For this review, take the finished solid that the model builds, in its own axes (mm). Face numbers are marked on the shaded views. A direction names the side the tool comes from. Round coordinates to 2 decimals unless told otherwise and drop trailing zeros. Write each loop counter-clockwise with the first axis right and the second up, starting at its lowest first coordinate (ties: lowest second). Pieces come first, ordered by that corner, then holes. Notation, with made-up numbers: (-10, 58) -> (20, 58) arc R13 cw to (20, 73) -> close; hole circle Ø3 at (-23.75, -12). An arc over 180 degrees is marked (long way). Answer in a Markdown table with one row per item.
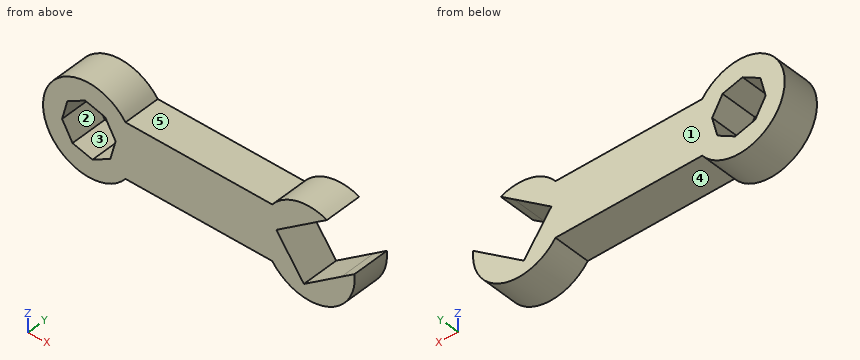
from build123d import *

# Parameters (mm, degrees)
F1_DEPTH = 25.4


with BuildPart() as f1:
    # F0 (on Front) → F1 (new body)
    with BuildSketch(Plane.XZ):
        with BuildLine():
            ThreePointArc((-50.790703, -19.05), (-46.070008, -10.040232), (-44.440703, 0))
            ThreePointArc((-44.440703, 0), (-46.070008, 10.040232), (-50.790703, 19.05))
            ThreePointArc((-50.790703, 19.05), (-107.940703, 0), (-50.790703, -19.05))
        make_face()
        Polygon((-78.729237, 18.529119), (-64.883652, 14.897081), (-57.661583, 2.538535), (-61.293621, -11.307051), (-73.652168, -18.529119), (-87.497754, -14.897081), (-94.719822, -2.538535), (-91.087784, 11.307051), align=None, mode=Mode.SUBTRACT)
        with BuildLine():
            ThreePointArc((-50.790703, 19.05), (-46.070008, 10.040232), (-44.440703, 0))
            ThreePointArc((-44.440703, 0), (-46.070008, -10.040232), (-50.790703, -19.05))
            Line((-50.790703, -19.05), (50.851671, -19.05))
            ThreePointArc((50.851671, -19.05), (44.501671, 0), (50.851671, 19.05))
            Line((50.851671, 19.05), (-50.790703, 19.05))
        make_face()
        with BuildLine():
            ThreePointArc((88.768213, 29.178737), (68.057545, 30.6744), (50.851671, 19.05))
            ThreePointArc((50.851671, 19.05), (44.501671, 0), (50.851671, -19.05))
            ThreePointArc((50.851671, -19.05), (87.767851, -29.587837), (107.846656, 3.133593))
            Line((107.846656, 3.133593), (98.813464, -3.48335))
            Line((98.813464, -3.48335), (72.76832, -22.561793))
            Line((72.76832, -22.561793), (53.689878, 3.48335))
            Line((53.689878, 3.48335), (79.735021, 22.561793))
            Line((79.735021, 22.561793), (88.768213, 29.178737))
        make_face()
    extrude(amount=F1_DEPTH)


solid = f1.part
1) Mouldability with a two-part tool opening along X and no side actions: class the marked faces 1 and 2 as pulls with the +X half, pulls with the -X half, needs draft (parallel to the pull), parting line crosses it, or undercut.
Solved:
| item | result |
|---|---|
| face 1 | needs draft |
| face 2 | undercut |
2) Consider section B-B on z = 0. State the section outline as (x, y) points.
Solved:
| item | result |
|---|---|
| outline | (-107.94, -25.4) -> (-94.05, -25.4) -> (-94.05, 0) -> (-107.94, 0) -> close; (-58.33, -25.4) -> (56.24, -25.4) -> (56.24, 0) -> (-58.33, 0) -> close; (103.57, -25.4) -> (108, -25.4) -> (108, 0) -> (103.57, 0) -> close |
3) Consider section C-C on x = -11.5. State the section outline as (y, z) points.
Solved:
| item | result |
|---|---|
| outline | (-25.4, -19.05) -> (0, -19.05) -> (0, 19.05) -> (-25.4, 19.05) -> close |
4) For the marked faces 3, 4 and 5, list the 3-axis set-ups (+Z, -Z, +X, -X, +Y, -Y) from which the entire face can be reached by the end or side of a thin tool; tool diameter is ignored.
Solved:
| item | result |
|---|---|
| face 3 | +Y, -Y |
| face 4 | -Z, +Y, -Y |
| face 5 | +Z, +Y, -Y |
5) Clearance check with flat-ended pins moving along their axes: pin 1 Ø12.5 at (x, y) = (19, -14.5) entering from +Z; pin 2 Ø12 at (y, z) = (-22.5, 24) entering from +X; pin 3 Ø1.5 at (y, z) = (-13, -5) entering from +X; pin 4 Ø3 at (x, y) = (75, -18) entering from -Z. State where each tip first meets the part, or that it passes through.
Solved:
| item | result |
|---|---|
| pin 1 | z = 19.05 |
| pin 2 | x = 88.77 |
| pin 3 | x = 107.72 |
| pin 4 | z = -31.75 |
6) Consider section A-A on y = -5.5. State the section outline as (x, z) points, then the cut area to 3 significant figures.
Solved:
| item | result |
|---|---|
| outline | (-50.79, -19.05) -> (50.85, -19.05) arc R31.75 ccw to (107.85, 3.13) -> (72.77, -22.56) -> (53.69, 3.48) -> (88.77, 29.18) arc R31.75 ccw to (50.85, 19.05) -> (-50.79, 19.05) arc R31.75 ccw (long way) to start; hole (-94.72, -2.54) -> (-87.5, -14.9) -> (-73.65, -18.53) -> (-61.29, -11.31) -> (-57.66, 2.54) -> (-64.88, 14.9) -> (-78.73, 18.53) -> (-91.09, 11.31) -> close |
| area | 7,390 mm² |
7) For line 1 (X direction, y = -2.5, z = 3); line 2 (X direction, y = -19, z = 0.5); line 3 (Z direction, x = -21.5, y = -12.5), list the stretches that pass through material, from the lowest coordinate up. Write a range as [from, to].
Solved:
| item | result |
|---|---|
| line 1 | [-107.8, -93.27], [-57.93, 54.04], [107.66, 107.86] |
| line 2 | [-107.94, -93.92], [-58.2, 55.88], [104.25, 108] |
| line 3 | [-19.05, 19.05] |
